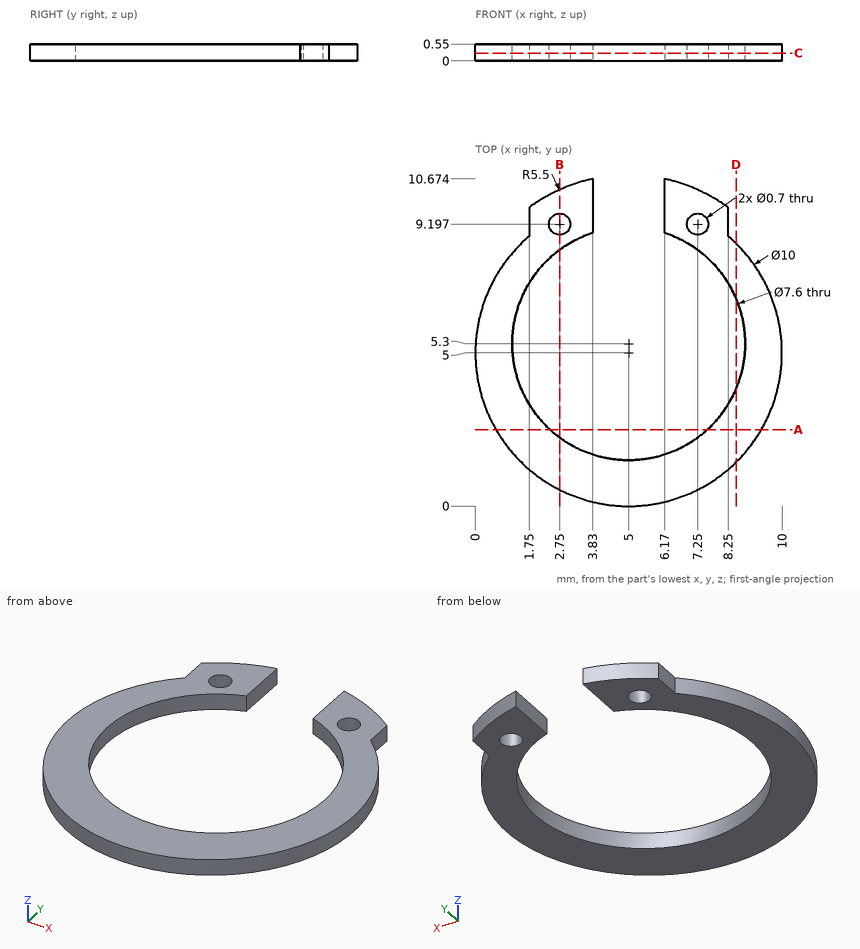
The drawing under review shows one solid part. Ordinate dimensions are in mm from its lowest x, y, z. Round coordinates to 2 decimals unless told otherwise and drop trailing zeros. Write each loop counter-clockwise with the first axis right and the second up, starting at its lowest first coordinate (ties: lowest second). Pieces come first, ordered by that corner, then holes.
(1) We need section A-A on y = 2.5. Give the boundary of the cut face in (x, z).
(2) We need section C-C on z = 0.25. Give the boundary of the cut face in (x, y).
(3) We need section D-D on x = 8.5. Give the boundary of the cut face in (y, z).
(4) Wall thickness on L1, parallel to Y at x = 2.75, z = 0.4 (1 decimal); L2, parallel to Y at x = 2.25, z = 0.45; L3, parallel to X at y = 5.3, z = 0.2: over which ranges is each line inside the solid? List them lowest first.
(5) Insertion check: pin 1 (1.5 mm diameter, centred on x = 2.5, y = 3, fed in from -Z); pin 2 (1.5 mm diameter, centred on x = 5, y = 9, fed in from -Z). Each pin has a flat end and moves straight along its axis. Give the tip position at first contact, or say it passes through.
(6) We need section B-B on x = 2.75. Give the number of separate pieces and of enclosed holes in the cut face, and give its area (3 significant figures).
Findings below:
1. outline: (0.67, 0) - (2.43, 0) - (2.43, 0.55) - (0.67, 0.55) - close; (7.57, 0) - (9.33, 0) - (9.33, 0.55) - (7.57, 0.55) - close
2. outline: (1.75, 8.8) arc R5 ccw (long way) to (8.25, 8.8) - (8.25, 9.74) arc R5.5 ccw to (6.17, 10.67) - (6.17, 8.92) arc R3.8 cw (long way) to (3.83, 8.92) - (3.83, 10.67) arc R5.5 ccw to (1.75, 9.74) - close; hole circle Ø0.7 at (2.75, 9.2); hole circle Ø0.7 at (7.25, 9.2)
3. outline: (1.43, 0) - (3.82, 0) - (3.82, 0.55) - (1.43, 0.55) - close; (6.78, 0) - (8.57, 0) - (8.57, 0.55) - (6.78, 0.55) - close
4. L1: y = 0.5 to 2.2, 8.4 to 8.8, 9.5 to 10.3
4. L2: y = 0.82 to 2.68, 7.92 to 10.06
4. L3: x = 0.01 to 1.2, 8.8 to 9.99
5. pin 1: stops at z = 0
5. pin 2: passes through
6. separate pieces: 3
6. enclosed holes: 0
6. area: 1.63 mm2
